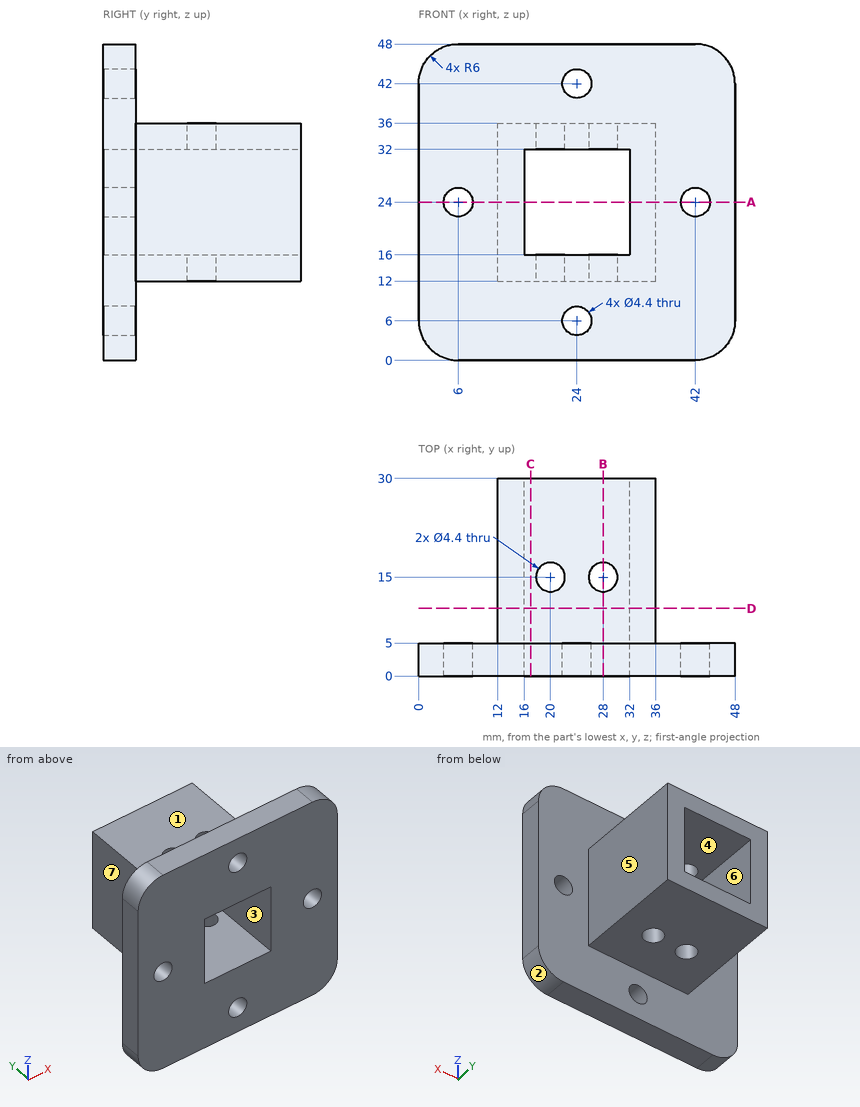
Verification items for this drawing (mm, ordinates from the low corner). A direction names the side the tool comes from. Round coordinates to 2 decimals unless told otherwise and drop trailing zeros. Loops run counter-clockwise (first coordinate to the right, second up) from the corner with the lowest first, then second, coordinate; pieces in that order, holes last. Notation, with made-up numbers: (62, -4.5) -> (91, -4.5) arc R8 ccw to (91, 2.5) -> close; hole circle Ø5 at (21, 75). An arc over 180 degrees is marked (long way). Answer in a Markdown table with one row per item.
Q1. Sectioned sample at C-C on x = 17. Enter the section's corners in (y, z).
Data:
| item | result |
|---|---|
| outline | (0, 0) -> (5, 0) -> (5, 12) -> (30, 12) -> (30, 16) -> (0, 16) -> close; (0, 32) -> (30, 32) -> (30, 36) -> (5, 36) -> (5, 48) -> (0, 48) -> close |
Q2. Release check for a two-part mould opening along X. For the marked faces 1, 2, 3 and 4 record: released by +X, released by -X, zero draft, split by the parting line, or undercut.
Data:
| item | result |
|---|---|
| face 1 | zero draft |
| face 2 | released by +X |
| face 3 | undercut |
| face 4 | undercut |
Q3. Sectioned sample at D-D on y = 10.25. Enter the section's corners in (x, z), then the cut area to 3 significant figures.
Data:
| item | result |
|---|---|
| outline | (12, 12) -> (36, 12) -> (36, 36) -> (12, 36) -> close; hole (16, 16) -> (32, 16) -> (32, 32) -> (16, 32) -> close |
| area | 320 mm^2 |
Q4. Set-up check for the marked faces 5, 6 and 7: record each of +Z, -Z, +X, -X, +Y, -Y from which the full face is reachable in a straight line by a thin tool's end or side.
Data:
| item | result |
|---|---|
| face 5 | +Z, -Z, +X, +Y |
| face 6 | +Y, -Y |
| face 7 | +Z, -Z, -X, +Y |
Q5. Sectioned sample at B-B on x = 28. Enter the section's corners in (y, z), then the cut area to 3 significant figures.
Data:
| item | result |
|---|---|
| outline | (0, 0) -> (5, 0) -> (5, 12) -> (12.8, 12) -> (12.8, 16) -> (0, 16) -> close; (0, 32) -> (12.8, 32) -> (12.8, 36) -> (5, 36) -> (5, 48) -> (0, 48) -> close; (17.2, 12) -> (30, 12) -> (30, 16) -> (17.2, 16) -> close; (17.2, 32) -> (30, 32) -> (30, 36) -> (17.2, 36) -> close |
| area | 325 mm^2 |
Q6. Go/stop test with flat-tipped pins: P1, Ø4, axis at x = 8, y = 3, coming from the -Z side; P2, Ø1, axis at x = 37.5, z = 28.5, coming from the +Y side; P3, Ø17.5, axis at x = 23.5, y = 16.5, coming from the +Z side; P4, Ø7, axis at y = 12, z = 22, coming from the +X side. Record where each tip stops, or that it passes through.
Data:
| item | result |
|---|---|
| P1 | stops at z = 0 |
| P2 | stops at y = 5 |
| P3 | stops at z = 36 |
| P4 | stops at x = 36 |
Q7. Thickness scan on L1, parallel to X at y = 15, z = 15.1; L2, parallel to X at y = 2.6, z = 24; L3, parallel to X at y = 3.3, z = 6. Record the ranges inside material, lowest first.
Data:
| item | result |
|---|---|
| L1 | x = 12 to 17.8, 22.2 to 25.8, 30.2 to 36 |
| L2 | x = 0 to 3.8, 8.2 to 16, 32 to 39.8, 44.2 to 48 |
| L3 | x = 0 to 21.8, 26.2 to 48 |
Q8. Sectioned sample at A-A on z = 24. Enter the section's corners in (x, y), then the cut area to 3 significant figures.
Data:
| item | result |
|---|---|
| outline | (0, 0) -> (3.8, 0) -> (3.8, 5) -> (0, 5) -> close; (8.2, 0) -> (16, 0) -> (16, 30) -> (12, 30) -> (12, 5) -> (8.2, 5) -> close; (32, 0) -> (39.8, 0) -> (39.8, 5) -> (36, 5) -> (36, 30) -> (32, 30) -> close; (44.2, 0) -> (48, 0) -> (48, 5) -> (44.2, 5) -> close |
| area | 316 mm^2 |
